The listing builds one solid part. Answer for the finished solid, in the listing's coordinates (mm). Face numbers are marked on the shaded views. Give positions to 0.01 mm unless a question says otherwise; leave off trailing zeros. Write each loop counter-clockwise with the first axis right and the second up, starting at its lowest first coordinate (ties: lowest second). Pieces come first, ordered by that corner, then holes. Notation, with made-up numbers: (63, 76.25) - (95, 76.25) arc R33 ccw to (95, 108.25) - close; hole circle Ø1 at (60.5, -32). An arc over 180 degrees is marked (long way). Return JSON: item names as keys, results as strings.
from build123d import *

# Parameters (mm, degrees)
F0_W                  = 152.4
F0_H                  = 63.5
F1_DEPTH              = 31.75
F3_D                  = 47.625
F5_D                  = 47.625
F10_W                 = 63.5
F10_H                 = 3.175
F11_DEPTH             = 19.05
F12_D                 = 7.9248
F12_CBORE_D           = 11.1252
F12_CBORE_DEPTH       = 31.75
F12_ON_F7_D           = 7.9248
F12_ON_F7_CBORE_D     = 11.1252
F12_ON_F7_CBORE_DEPTH = 31.75
F12_ON_F8_D           = 7.9248
F12_ON_F8_CBORE_D     = 11.1252
F12_ON_F8_CBORE_DEPTH = 31.75
F12_ON_F9_D           = 7.9248
F12_ON_F9_CBORE_D     = 11.1252
F12_ON_F9_CBORE_DEPTH = 31.75
F13_W                 = 6.35
F13_H                 = 63.5
F14_DEPTH             = 50.8


with BuildPart() as f1:
    # F0 (on Front) → F1 (new body, symmetric)
    with BuildSketch(Plane.XZ):
        Rectangle(F0_W, F0_H)
    extrude(amount=F1_DEPTH, both=True)

    # F3 (through all)
    with Locations(Plane.XY.offset(31.75)):
        with Locations((-34.925, 0)):
            Hole(F3_D / 2)

    # F5 (through all)
    with Locations(Plane.XZ.offset(31.75)):
        with Locations((34.925, 0)):
            Hole(F5_D / 2)

    # F10 (on face) → F11 (cut, symmetric)
    with BuildSketch(Plane.YZ.offset(76.2)):
        Rectangle(F10_W, F10_H)
    extrude(amount=F11_DEPTH, both=True, mode=Mode.SUBTRACT)

    # F12 (through all)
    with Locations(Plane.XY.offset(31.75)):
        with Locations((66.675, 19.05)):
            CounterBoreHole(F12_D / 2, F12_CBORE_D / 2, F12_CBORE_DEPTH)

    # F12 on F7 (through all)
    with Locations(Plane.XY.offset(31.75)):
        with Locations((66.675, -19.05)):
            CounterBoreHole(F12_ON_F7_D / 2, F12_ON_F7_CBORE_D / 2, F12_ON_F7_CBORE_DEPTH)

    # F12 on F8 (through all)
    with Locations(Plane.XZ.offset(31.75)):
        with Locations((-66.675, 19.05)):
            CounterBoreHole(F12_ON_F8_D / 2, F12_ON_F8_CBORE_D / 2, F12_ON_F8_CBORE_DEPTH)

    # F12 on F9 (through all)
    with Locations(Plane.XZ.offset(31.75)):
        with Locations((-66.675, -21.2032347918)):
            CounterBoreHole(F12_ON_F9_D / 2, F12_ON_F9_CBORE_D / 2, F12_ON_F9_CBORE_DEPTH)

    # F13 (on face) → F14 (cut)
    with BuildSketch(Plane(origin=(-76.2, 0, 0), x_dir=(0, -1, 0), z_dir=(-1, 0, 0))):
        Rectangle(F13_W, F13_H)
    extrude(amount=-F14_DEPTH, mode=Mode.SUBTRACT)


solid = f1.part
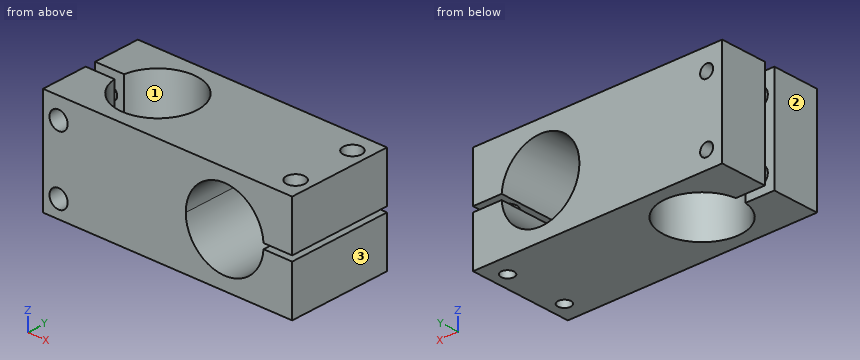
Item 1: The mould has two halves that part along X. Classify the marked faces 1, 2 and 3: +X half, -X half, draft (parallel to the pull), parting line (faces both ways), or undercut.
Answer below:
{"face 1": "undercut", "face 2": "-X half", "face 3": "+X half"}
Item 2: A flat-ended cylindrical pin translates along its axis: P1, Ø6.5, axis at x = -66.675, z = 19.05, coming from the +Y side. Find the tip coordinate at first contact, or state that the pin passes through.
Answer below:
{"P1": "passes through"}
Item 3: A cutting plane is placed at D-D on x = -21. Determine the outline of the cut face in (y, z).
Answer below:
{"outline": "(-31.75, -31.75) - (-19.32, -31.75) - (-19.32, 31.75) - (-31.75, 31.75) - close; (19.32, -31.75) - (31.75, -31.75) - (31.75, 31.75) - (19.32, 31.75) - close"}
Item 4: A cutting plane is placed at A-A on y = 10. Give the number of separate pieces and of enclosed holes in the cut face, then the cut area to 3 significant figures.
Answer below:
{"separate pieces": "2", "enclosed holes": "2", "area": "5,000 mm²"}
Item 5: Consider L1, parallel to Y at x = -62.5, z = -6 (3 decimals); L2, parallel to X at y = -24, z = 19; L3, parallel to Y at x = 68, z = -6.5. Determine where each line is inside the solid, lowest interval first.
Answer below:
{"L1": "y = -31.75 to -3.175, 3.175 to 31.75", "L2": "x = -76.2 to -72.24, -61.11 to 20.57, 49.28 to 64.14, 69.21 to 76.2", "L3": "y = -31.75 to -22.78, -15.32 to 15.32, 22.78 to 31.75"}
